Autodesk Inventor part; units mm, degrees
ref_plane "YZ Plane" through (0, 0, 0) normal (1, 0, 0) x (0, 1, 0)
ref_plane "XZ Plane" through (0, 0, 0) normal (0, 1, 0) x (-1, 0, 0)
ref_plane "XY Plane" through (0, 0, 0) normal (0, 0, 1) x (1, 0, 0)
sketch "Sketch1" plane through (0, 0, 0) normal (0, 1, 0) x (-1, 0, 0)
  line L0 (0, 0) -> (107, 0)
  line L1 (107, 0) -> (107, -124)
  line L2 (107, -124) -> (0, -124)
  line L3 (0, -124) -> (0, 0)
  point P0 (53.5, -124)
  dimension "d0" = 107
  dimension "d1" = 124
extrude "Plate1" add sketch "Sketch1" along normal blind 3
sketch "Sketch2" plane through (-3, 0, -124) normal (1, 0, 0) x (0, 1, 0)
  line L0 (0, 124) -> (0, 0)
  line L1 (0, 0) -> (107, 0)
  line L2 (107, 0) -> (107, 124)
  line L3 (107, 124) -> (0, 124)
edge flange "Flange1" height 107 angle 90 thickness 3 bend radius 3 thickness toward (1, 0, 0) relief tear relief width 3 relief depth 1.5 edges at (0, 3, -62) wall of the first edge with corners at (-3, 0, 0) (-3, 0, -124) (-3, 107, -124) (-3, 107, 0)
bend "Bend1"
corner "Corner1"
sketch "Sketch6" plane through (0, 0, 0) normal (0, -1, 0) x (1, 0, 0)
  circle A0 centre (-78, -118) radius 1.75
  line L0 (-107, -124) -> (-107, 0)
  line L1 (-6, -124) -> (-107, -124)
  circle A1 centre (-78, -34.5) radius 1.75
  circle A2 centre (-17.5, -118) radius 1.75
  circle A3 centre (-17.5, -34.5) radius 1.75
  circle A4 centre (-78, -6) radius 1.75
  line L2 (-107, 0) -> (-6, 0)
  circle A5 centre (-78, -89.5) radius 1.75
  circle A6 centre (-17.5, -6) radius 1.75
  circle A7 centre (-17.5, -89.5) radius 1.75
  point P0 (0, 0)
  dimension "d79" = 3.5
  dimension "d80" = 29
  dimension "d81" = 6
  dimension "d84" = 83.5
  dimension "d87" = 60.5
  dimension "d113" = 3.5
  dimension "d114" = 6
  dimension "d115" = 29
  dimension "d118" = 83.5
  dimension "d121" = 60.5
extrude "Cut4" cut sketch "Sketch6" against normal blind 3
sketch "Sketch7" plane through (0, 107, 0) normal (1, 0, 0) x (0, 0, -1)
  line L0 (120, -84) -> (116, -84)
  line L1 (116, -84) -> (116, -94)
  line L2 (116, -94) -> (120, -94)
  line L3 (120, -94) -> (120, -84)
  line L4 (124, 0) -> (124, -101)
  line L5 (124, -107) -> (0, -107)
  line L6 (120, -10) -> (116, -10)
  line L7 (116, -10) -> (116, -20)
  line L8 (116, -20) -> (120, -20)
  line L9 (120, -20) -> (120, -10)
  line L10 (8, -84) -> (4, -84)
  line L11 (4, -84) -> (4, -94)
  line L12 (4, -94) -> (8, -94)
  line L13 (8, -94) -> (8, -84)
  line L14 (8, -10) -> (4, -10)
  line L15 (4, -10) -> (4, -20)
  line L16 (4, -20) -> (8, -20)
  line L17 (8, -20) -> (8, -10)
  point P0 (124, -27)
  point P1 (124, -33)
  point P2 (12, -101)
  point P3 (12, -107)
  point P4 (12, -27)
  point P5 (12, -33)
  dimension "d92" = 10
  dimension "d93" = 4
  dimension "d94" = 4
  dimension "d95" = 13
  dimension "d105" = 74
  dimension "d108" = 112
extrude "Extrusion1" cut sketch "Sketch7" against normal blind 3
equation "\"d114\" = d81"
equation "\"d115\" = d80"
equation "\"d118\" = d84"
equation "\"d121\" = d87"
equation "\"d90\" = Thickness"
equation "\"d108\" = d1 - d93 - 2 * d94"
equation "\"d24\" = Thickness"
equation "\"d25\" = BendReliefWidth"
equation "\"d26\" = BendReliefDepth"
equation "\"d27\" = MinimumRemnant"
equation "\"d28\" = TransitionRadius"
equation "\"d29\" = d0"
equation "\"d31\" = BendRadius"
equation "\"d32\" = CornerReliefSize"
equation "\"d33\" = GapSize"
equation "\"d34\" = JacobiRadiusSize"
equation "\"BendRadius\" = Thickness"
equation "\"BendReliefWidth\" = Thickness"
equation "\"BendReliefDepth\" = 0.5 * Thickness"
equation "\"CornerReliefSize\" = 4 * Thickness"
equation "\"MinimumRemnant\" = 2 * Thickness"
equation "\"TransitionRadius\" = BendRadius"
equation "\"JacobiRadiusSize\" = BendRadius"
equation "\"GapSize\" = Thickness"
properties part number "Face with CWT hole" material "Steel, Carbon"
Part model, mm, in its own coordinate system. A direction names the side the tool comes from. Round coordinates to 2 decimals unless told otherwise and drop trailing zeros. Order: outer loops, then holes, each group sorted by start corner. A loop starts at its lowest first (then second) coordinate and runs counter-clockwise, first axis right, second up. Notation, with made-up numbers: M 67.25,11 L 102.25,11 A25 cw 102.25,26 Z; hole C 12,-33 d11. An arc over 180 degrees is marked long. Put each result on its own line as item: value. Start each with the question number.
1. Drop flat-ended pins along their axis: pin 1 (6 mm diameter, centred on y = 76, z = -15, fed in from -X); pin 2 (1 mm diameter, centred on x = -17, z = -46, fed in from +Y); pin 3 (1.5 mm diameter, centred on x = -1.5, z = -6.5, fed in from -Y). Give the stop position or say it passes through.
2. Slice it at C-C on x = -91. List the corners of the cut face in (y, z).
3. Two-plate mould, pull along Z, no slides. Class faces 3 (the face through (-1, 97, -6)), 4 (the face through (-56, 3, -61)): +Z half, -Z half, draft (parallel to the pull), parting line (faces both ways), or undercut.
4. Slice it at B-B on z = -34.5. List the corners of the cut face in (x, y).
5. Tool access for faces 1 (the face through (-1, 87, -6)), 2 (the face through (-19.25, 1.48, -34.42)): list every direction of +Z, -Z, +X, -X, +Y, -Y with a clear straight run to the whole face (end or side of a thin tool).
6. Slice it at A-A on z = -118. List the corners of the cut face in (x, y).
7. Drill centre lines: probe 1 along Z at (x, y) = (-78, 2.4); probe 2 along Y at (x, z) = (-22, -110); probe 3 along X at (y, z) = (101, -41). Where is each one in solid material? Low to high. Write a range as [from, to].
8. Slice it at D-D on y = 48.5. List the corners of the cut face in (x, z).
Findings:
1. pin 1: x = -3
1. pin 2: y = 3
1. pin 3: y = 1.32
2. outline: M 0,-124 L 3,-124 L 3,0 L 0,0 Z
3. face 3: undercut
3. face 4: draft
4. outline: M -107,0 L -79.75,0 L -79.75,3 L -107,3 Z; M -76.25,0 L -19.25,0 L -19.25,3 L -76.25,3 Z; M -15.75,0 L -6,0 A6 ccw 0,6 L 0,107 L -3,107 L -3,6 A3 cw -6,3 L -15.75,3 Z
5. face 1: +X, -X
5. face 2: +Y, -Y
6. outline: M -107,0 L -79.75,0 L -79.75,3 L -107,3 Z; M -76.25,0 L -19.25,0 L -19.25,3 L -76.25,3 Z; M -15.75,0 L -6,0 A6 ccw 0,6 L 0,13 L -3,13 L -3,6 A3 cw -6,3 L -15.75,3 Z; M -3,23 L 0,23 L 0,87 L -3,87 Z; M -3,97 L 0,97 L 0,107 L -3,107 Z
7. probe 1: [-124, -119.75], [-116.25, -91.25], [-87.75, -36.25], [-32.75, -7.75], [-4.25, 0]
7. probe 2: [0, 3]
7. probe 3: [-3, 0]
8. outline: M -3,-124 L 0,-124 L 0,0 L -3,0 Z
